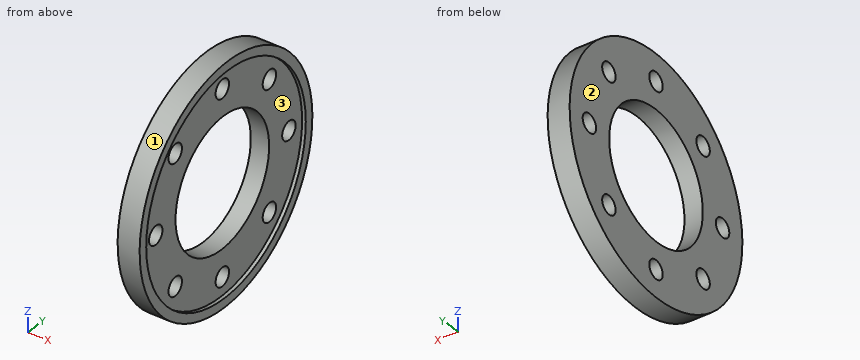
from build123d import *

# Parameters (mm, degrees)
SKETCH_1_R           = 65.5
SKETCH_1_R_2         = 35.5
SKETCH_1_R_3         = 5.1
EXTRUDE_1_DEPTH      = 6
SKETCH_2_OUTSIDE_W   = 170.13
SKETCH_2_OUTSIDE_H   = 170.13
SKETCH_2_OUTSIDE_R   = 65.5
SKETCH_2_OUTSIDE_R_2 = 60.5
CUT_EXTRUDE_1_DEPTH  = 2


with BuildPart() as part:
    # Эскиз1 → Бобышка-Вытянуть1 (new, symmetric)
    with BuildSketch(Plane(origin=(0, 0, 0), x_dir=(0, 0, -1), z_dir=(1, 0, 0))):
        Circle(SKETCH_1_R)
        Circle(SKETCH_1_R_2, mode=Mode.SUBTRACT)
        with Locations((0, 50.5)):
            Circle(SKETCH_1_R_3, mode=Mode.SUBTRACT)
        with Locations((35.70889245, 35.70889245)):
            Circle(SKETCH_1_R_3, mode=Mode.SUBTRACT)
        with Locations((50.5, 0)):
            Circle(SKETCH_1_R_3, mode=Mode.SUBTRACT)
        with Locations((35.70889245, -35.70889245)):
            Circle(SKETCH_1_R_3, mode=Mode.SUBTRACT)
        with Locations((0, -50.5)):
            Circle(SKETCH_1_R_3, mode=Mode.SUBTRACT)
        with Locations((-35.70889245, -35.70889245)):
            Circle(SKETCH_1_R_3, mode=Mode.SUBTRACT)
        with Locations((-50.5, 0)):
            Circle(SKETCH_1_R_3, mode=Mode.SUBTRACT)
        with Locations((-35.70889245, 35.70889245)):
            Circle(SKETCH_1_R_3, mode=Mode.SUBTRACT)
    extrude(amount=EXTRUDE_1_DEPTH, both=True)

    # Эскиз2 outside → Вырез-Вытянуть1 (cut)
    # profile 1 of 2: a face of its own
    with BuildSketch(Plane(origin=(6, 0, 0), x_dir=(0, 0, -1), z_dir=(1, 0, 0))):
        Rectangle(SKETCH_2_OUTSIDE_W, SKETCH_2_OUTSIDE_H)
        Circle(SKETCH_2_OUTSIDE_R, mode=Mode.SUBTRACT)
    # profile 2 of 2: a face of its own
    with BuildSketch(Plane(origin=(6, 0, 0), x_dir=(0, 0, -1), z_dir=(1, 0, 0))):
        Circle(SKETCH_2_OUTSIDE_R_2)
    extrude(amount=-CUT_EXTRUDE_1_DEPTH, mode=Mode.SUBTRACT)


solid = part.part
Part model, mm, in its own coordinate system. Face numbers are marked on the shaded views. Coordinates: 2 decimals unless noted, no trailing zeros. Order: outer loops, then holes, each group sorted by start corner. A loop starts at its lowest first (then second) coordinate and runs counter-clockwise, first axis right, second up.
(1) Pin check, flat tips, straight feed: pin 1 Ø3 at (y, z) = (-1.5, 52) entering from +X; pin 2 Ø3 at (x, y) = (0.5, -44) entering from +Z; pin 3 Ø4 at (x, z) = (4.5, 32) entering from -Y; pin 4 Ø13.5 at (y, z) = (50.5, 0) entering from +X. Stop position of each tip, or through.
Check sheet entries:
pin 1: passes through
pin 2: stops at z = 49.84
pin 3: stops at y = -58.23
pin 4: stops at x = 4
(2) Pull direction Z, two halves, no side cores. Call the marked faces 1, 2 and 3: pulls with the +Z half, pulls with the -Z half, needs draft (parallel to the pull), parting line crosses it, or undercut.
Check sheet entries:
face 1: parting line crosses it
face 2: needs draft
face 3: undercut
(3) Slice it at A-A, the plane y = 0. Write the cut outline in (x, z).
Check sheet entries:
outline: (-6, -65.5) - (6, -65.5) - (6, -60.5) - (4, -60.5) - (4, -55.6) - (-6, -55.6) - close; (-6, -45.4) - (4, -45.4) - (4, -35.5) - (-6, -35.5) - close; (-6, 35.5) - (4, 35.5) - (4, 45.4) - (-6, 45.4) - close; (-6, 55.6) - (4, 55.6) - (4, 60.5) - (6, 60.5) - (6, 65.5) - (-6, 65.5) - close
(4) Slice it at D-D, the plane x = -1. State how many separate pieces and enclosed holes the cut face has, and give its area (3 significant figures).
Check sheet entries:
separate pieces: 1
enclosed holes: 9
area: 8,870 mm2
(5) Probe L1, parallel to Y at x = -1, z = 0; L2, parallel to Z at x = 3, y = -0.5; L3, parallel to Y at x = -5, z = -4.5. List the from-to ranges inside material, lowest first.
Check sheet entries:
L1: y = -65.5 to -55.6, -45.4 to -35.5, 35.5 to 45.4, 55.6 to 65.5
L2: z = -65.5 to -55.58, -45.42 to -35.5, 35.5 to 45.42, 55.58 to 65.5
L3: y = -65.35 to -52.9, -48.1 to -35.21, 35.21 to 48.1, 52.9 to 65.35
(6) Slice it at C-C, the plane z = -50.5. Write the cut outline in (x, y), and give its area (3 significant figures).
Check sheet entries:
outline: (-6, -41.71) - (6, -41.71) - (6, -33.32) - (4, -33.32) - (4, -5.1) - (-6, -5.1) - close; (-6, 5.1) - (4, 5.1) - (4, 33.32) - (6, 33.32) - (6, 41.71) - (-6, 41.71) - close
area: 766 mm2
